Geometry check sheet. Reference: drawing and pictorial views, mm from the part's lowest x, y, z. Give positions to 0.01 mm unless a question says otherwise; leave off trailing zeros. Write each loop counter-clockwise with the first axis right and the second up, starting at its lowest first coordinate (ties: lowest second). Pieces come first, ordered by that corner, then holes. Notation, with made-up numbers: M 65,72 L 86,72 A16 ccw 86,103 Z; hole C 43.25,83 d4. An arc over 180 degrees is marked long. Answer as a JSON object with one key per item and string values.
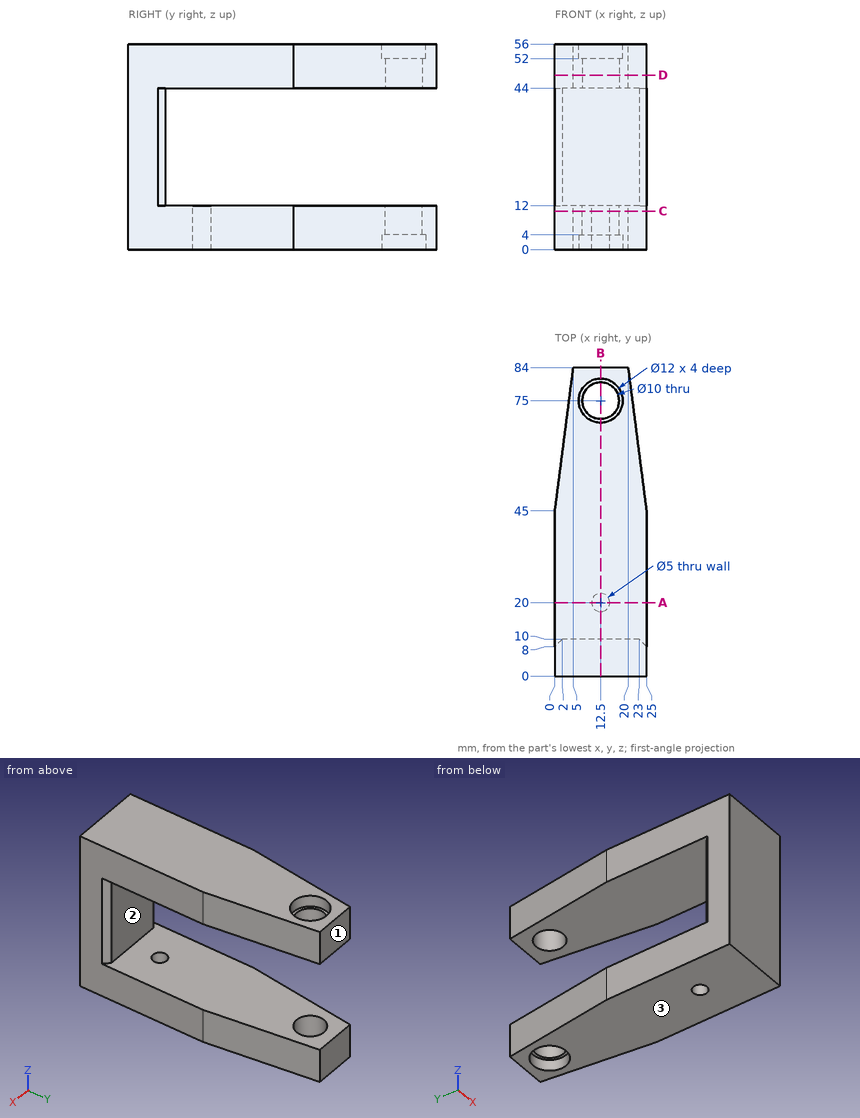
1) Go/stop test with flat-tipped pins: pin 1 (1 mm diameter, centred on x = 20, z = 32, fed in from -Y); pin 2 (3.5 mm diameter, centred on x = 15.5, y = 73.5, fed in from +Z); pin 3 (10.5 mm diameter, centred on x = 12, z = 22.5, fed in from +Y). Record where each tip stops, or that it passes through.
Completed:
{"pin 1": "stops at y = 0", "pin 2": "stops at z = 52", "pin 3": "stops at y = 10"}
2) Section check D-D on z = 47.5. Record the boundary of the cut face in (x, y), and give its area (3 significant figures).
Completed:
{"outline": "M 0,0 L 25,0 L 25,45 L 20,84 L 5,84 L 0,45 Z; hole C 12.5,75 d10", "area": "1,830 mm2"}
3) Section check A-A on y = 20. Record the boundary of the cut face in (x, z).
Completed:
{"outline": "M 0,0 L 10,0 L 10,12 L 0,12 Z; M 0,44 L 25,44 L 25,56 L 0,56 Z; M 15,0 L 25,0 L 25,12 L 15,12 Z"}
4) Section check B-B on x = 12.5. Record the boundary of the cut face in (y, z), and give its area (3 significant figures).
Completed:
{"outline": "M 0,0 L 17.5,0 L 17.5,12 L 10,12 L 10,44 L 70,44 L 70,52 L 69,52 L 69,56 L 0,56 Z; M 22.5,0 L 69,0 L 69,4 L 70,4 L 70,12 L 22.5,12 Z; M 80,4 L 81,4 L 81,0 L 84,0 L 84,12 L 80,12 Z; M 80,44 L 84,44 L 84,56 L 81,56 L 81,52 L 80,52 Z", "area": "2,020 mm2"}
5) Thickness scan on L1, parallel to Y at x = 12.5, z = 2.1; L2, parallel to Z at x = 6.25, y = 77; L3, parallel to Y at x = 12.5, z = 54.75. Record the ranges inside material, lowest first.
Completed:
{"L1": "y = 0 to 17.5, 22.5 to 69, 81 to 84", "L2": "z = 0 to 12, 44 to 56", "L3": "y = 0 to 69, 81 to 84"}
6) Section check C-C on z = 10.5. Record the boundary of the cut face in (x, y).
Completed:
{"outline": "M 0,0 L 25,0 L 25,45 L 20,84 L 5,84 L 0,45 Z; hole C 12.5,75 d10; hole C 12.5,20 d5"}
7) Release check for a two-part mould opening along Z. For the marked faces 1, 2 and 3 record: pulls with the +Z half, pulls with the -Z half, needs draft (parallel to the pull), parting line crosses it, or undercut.
Completed:
{"face 1": "needs draft", "face 2": "undercut", "face 3": "pulls with the -Z half"}
